Could you check a few things on this model? Use its own coordinates, in mm. Face numbers are marked on the shaded views. A direction names the side the tool comes from. Round coordinates to 2 decimals unless told otherwise and drop trailing zeros. Loops run counter-clockwise (first coordinate to the right, second up) from the corner with the lowest first, then second, coordinate; pieces in that order, holes last. Notation, with made-up numbers: M 5,33 L 12,33 A19 cw 12,38 Z; hole C 32.25,21 d11. An arc over 180 degrees is marked long. One line per item, written item: value. Start each with the question number.
Q1. Which directions (+Z, -Z, +X, -X, +Y, -Y) give clear straight access to the entire face, cutting with the end or side of a thin tool? Please do the marked faces 1, 2 and 3.
Q2. Imagine slicing it at B-B (z = -8). Please give me the cut outline in (x, y).
Q3. I'm going to push flat-ended pins straight in: pin 1 Ø4 at (x, y) = (-72.86, 11.88) entering from -Z (1 decimal); pin 2 Ø4 at (x, z) = (-1, 0.5) entering from -Y; pin 3 Ø6 at (x, y) = (-41.11, 11.88) entering from -Z; pin 4 Ø1 at (y, z) = (0, 17) entering from -X. Where does each tip first touch, or does it pass through?
Q4. Please list where these lines run through material, in increasing order: line 1 along X through (y, z) = (-2.75, -8); line 2 along X through (y, z) = (-2, 0); line 3 along Y through (x, z) = (-7, 3).
Q5. Imagine slicing it at C-C (y = 15.5). Please give me the cut outline in (x, z), then the cut area to 3 significant figures.
Q6. Imagine slicing it at D-D (x = -62.5). Please give me the cut outline in (y, z) (3 decimals), then the cut area to 3 significant figures.
Q7. Imagine slicing it at A-A (y = -4). Give the number of separate pieces and of enclosed holes in the cut face, then the cut area to 3 significant figures.
from build123d import *

# Parameters (mm, degrees)
SKETCH6_W                = 9.525
SKETCH6_H                = 25.4
BOSS_EXTRUDE1_DEPTH      = 8
SKETCH16_W               = 8
SKETCH16_H               = 23
BOSS_EXTRUDE6_DEPTH      = 8
SKETCH7_R                = 3
SKETCH7_R_2              = 2.4
CUT_EXTRUDE1_DEPTH       = 0.8
SKETCH7_3_R              = 2.4
CUT_EXTRUDE2_DEPTH       = 7.2
SKETCH9_R                = 3
CUT_EXTRUDE4_DEPTH       = 0.8
BOSS_EXTRUDE3_DEPTH      = 8
FILLET1_R                = 3.175
FILLET3_R                = 3.175
BOSS_EXTRUDE7_DEPTH      = 18.225
BOSS_EXTRUDE7_DEPTH_BACK = 26.225
SKETCH18_W               = 44.45
SKETCH18_H               = 6.35
FILLET6_R                = 12.7
FILLET7_R                = 6.35
SKETCH11_W               = 8
SKETCH11_H               = 23
BOSS_EXTRUDE4_DEPTH      = 6.746167864
SKETCH14_W               = 8
SKETCH14_H               = 23
BOSS_EXTRUDE5_DEPTH      = 3.6
SKETCH13_R               = 3.1
SKETCH13_R_2             = 2.4
CUT_EXTRUDE5_DEPTH       = 0.8
CUT_EXTRUDE6_START       = -8
CUT_EXTRUDE6_OUTLINE_R   = 2.4
CUT_EXTRUDE6_DEPTH       = 8
F_8_CLEARANCE_HOLE1_D    = 4.4958
FILLET8_R                = 3.175


# Read off the part's stored shape, not the designer's step: Cut-Extrude6
with BuildPart() as part:
    # Sketch6 → Boss-Extrude1 (new body)
    with BuildSketch(Plane(origin=(0, 0, 0), x_dir=(1, 0, 0), z_dir=(0, 1, 0))):
        Rectangle(SKETCH6_W, SKETCH6_H)
    extrude(amount=-BOSS_EXTRUDE1_DEPTH)

    # Sketch16 → Boss-Extrude6 (add)
    with BuildSketch(Plane.XZ):
        with Locations((-6.442250006, 5.512369214)):
            Rectangle(SKETCH16_W, SKETCH16_H)
    extrude(amount=BOSS_EXTRUDE6_DEPTH)

    # Sketch7 → Cut-Extrude1 (cut)
    # profile 1 of 3: a face of its own
    with BuildSketch(Plane(origin=(0, 0, 0), x_dir=(1, 0, 0), z_dir=(0, 1, 0))):
        with Locations(Location((0, 8, 0), (0, 0, 270))):
            Circle(SKETCH7_R)
        with Locations(Location((0, 8, 0), (0, 0, 270))):
            Circle(SKETCH7_R_2, mode=Mode.SUBTRACT)
    # profile 2 of 3: a face of its own
    with BuildSketch(Plane(origin=(0, 0, 0), x_dir=(1, 0, 0), z_dir=(0, 1, 0))):
        with Locations(Location((0, 0, 0), (0, 0, 270))):
            Circle(SKETCH7_R)
        with Locations(Location((0, 0, 0), (0, 0, 270))):
            Circle(SKETCH7_R_2, mode=Mode.SUBTRACT)
    # profile 3 of 3: a face of its own
    with BuildSketch(Plane(origin=(0, 0, 0), x_dir=(1, 0, 0), z_dir=(0, 1, 0))):
        with Locations(Location((0, -8, 0), (0, 0, 270))):
            Circle(SKETCH7_R)
        with Locations(Location((0, -8, 0), (0, 0, 270))):
            Circle(SKETCH7_R_2, mode=Mode.SUBTRACT)
    extrude(amount=-CUT_EXTRUDE1_DEPTH, mode=Mode.SUBTRACT)

    # Sketch7<3> → Cut-Extrude2 (cut)
    with BuildSketch(Plane(origin=(0, 0, 0), x_dir=(1, 0, 0), z_dir=(0, 1, 0))):
        with Locations(Location((0, 8, 0), (0, 0, 270))):
            Circle(SKETCH7_3_R)
        with Locations(Location((0, 0, 0), (0, 0, 270))):
            Circle(SKETCH7_3_R)
        with Locations(Location((0, -8, 0), (0, 0, 270))):
            Circle(SKETCH7_3_R)
    extrude(amount=-CUT_EXTRUDE2_DEPTH, mode=Mode.SUBTRACT)

    # Sketch9 → Cut-Extrude4 (cut)
    with BuildSketch(Plane(origin=(0, -7.2, -7.2), x_dir=(1, 0, 0), z_dir=(0, 1, 0))):
        with Locations(Location((0, 0.8, 0), (0, 0, 270))):
            Circle(SKETCH9_R)
        with Locations(Location((0, -7.2, 0), (0, 0, 270))):
            Circle(SKETCH9_R)
        with Locations(Location((0, -15.2, 0), (0, 0, 270))):
            Circle(SKETCH9_R)
    extrude(amount=-CUT_EXTRUDE4_DEPTH, mode=Mode.SUBTRACT)

    # Sketch10 → Boss-Extrude3 (add)
    with BuildSketch(Plane(origin=(0, -8, 0), x_dir=(-1, 0, 0), z_dir=(0, -1, 0))):
        Polygon((4.7625, 4.223850374), (34.7625, -22.098), (60.1625, -22.098), (60.1625, -28.448), (32.37167179, -28.448), (4.7625, -4.223850374), align=None)
    extrude(amount=-BOSS_EXTRUDE3_DEPTH)

    # Fillet1
    fillet1_edges = [part.edges().sort_by_distance(p)[0] for p in [
        (-2.442250006, -4, 12.7),
        (-4.7625, -4, -5.987630786),
    ]]
    fillet(fillet1_edges, radius=FILLET1_R)

    # Fillet3
    fillet3_edges = [part.edges().sort_by_distance(p)[0] for p in [
        (4.7625, -4, 12.7),
        (-4.7625, -4, -12.7),
        (4.7625, -4, -12.7),
    ]]
    fillet(fillet3_edges, radius=FILLET3_R)

    # Sketch18 → Boss-Extrude7 (add, two sides: drawn at the far end of the back side and taken through both)
    with BuildSketch(Plane(origin=(0, 0, 0), x_dir=(1, 0, 0), z_dir=(0, 1, 0)).offset(-BOSS_EXTRUDE7_DEPTH_BACK)):
        with Locations((-56.9875, -25.273)):
            Rectangle(SKETCH18_W, SKETCH18_H)
    extrude(amount=BOSS_EXTRUDE7_DEPTH + BOSS_EXTRUDE7_DEPTH_BACK)

    # Fillet6
    fillet6_edges = [part.edges().sort_by_distance(p)[0] for p in [
        (-32.37167179, -4, 28.448),
    ]]
    fillet(fillet6_edges, radius=FILLET6_R)

    # Fillet7
    fillet7_edges = [part.edges().sort_by_distance(p)[0] for p in [
        (-34.7625, -4, 22.098),
    ]]
    fillet(fillet7_edges, radius=FILLET7_R)

    # Sketch11 → Boss-Extrude4 (add)
    with BuildSketch(Plane(origin=(0, -8, 0), x_dir=(-1, 0, 0), z_dir=(0, -1, 0))):
        with Locations((6.44225, -5.512369144)):
            Rectangle(SKETCH11_W, SKETCH11_H)
    extrude(amount=BOSS_EXTRUDE4_DEPTH)

    # Sketch14 → Boss-Extrude5 (add)
    with BuildSketch(Plane(origin=(0, -14.746167864, 0), x_dir=(-1, 0, 0), z_dir=(0, -1, 0))):
        with Locations((6.44225, -5.512369144)):
            Rectangle(SKETCH14_W, SKETCH14_H)
    extrude(amount=BOSS_EXTRUDE5_DEPTH)

    # Sketch13 → Cut-Extrude5 (cut)
    # profile 1 of 3: a face of its own
    with BuildSketch(Plane(origin=(-2.442250006, 0, 0), x_dir=(0, 0, -1), z_dir=(1, 0, 0))):
        with Locations((-13.512369144, -14.746167864)):
            Circle(SKETCH13_R)
        with Locations((-13.512369144, -14.746167864)):
            Circle(SKETCH13_R_2, mode=Mode.SUBTRACT)
    # profile 2 of 3: a face of its own
    with BuildSketch(Plane(origin=(-2.442250006, 0, 0), x_dir=(0, 0, -1), z_dir=(1, 0, 0))):
        with Locations((2.487630856, -14.746167864)):
            Circle(SKETCH13_R)
        with Locations((2.487630856, -14.746167864)):
            Circle(SKETCH13_R_2, mode=Mode.SUBTRACT)
    # profile 3 of 3: a face of its own
    with BuildSketch(Plane(origin=(-2.442250006, 0, 0), x_dir=(0, 0, -1), z_dir=(1, 0, 0))):
        with BuildLine():
            Line((-6.312369144, -14.014797014), (-6.312369144, -12.552055314))
            ThreePointArc((-6.312369144, -12.552055314), (-5.512369144, -12.425918689), (-4.712369144, -12.552055314))
            Line((-4.712369144, -12.552055314), (-4.712369144, -14.014797014))
            Line((-4.712369144, -14.014797014), (-3.249627444, -14.014797014))
            ThreePointArc((-3.249627444, -14.014797014), (-3.144641809, -14.746167864), (-3.249627444, -15.477538714))
            Line((-3.249627444, -15.477538714), (-4.712369144, -15.477538714))
            Line((-4.712369144, -15.477538714), (-4.712369144, -16.940280414))
            ThreePointArc((-4.712369144, -16.940280414), (-5.512369144, -17.066417039), (-6.312369144, -16.940280414))
            Line((-6.312369144, -16.940280414), (-6.312369144, -15.477538714))
            Line((-6.312369144, -15.477538714), (-7.775110844, -15.477538714))
            ThreePointArc((-7.775110844, -15.477538714), (-7.880096479, -14.746167864), (-7.775110844, -14.014797014))
            Line((-7.775110844, -14.014797014), (-6.312369144, -14.014797014))
        make_face()
    cut_extrude5 = extrude(amount=-CUT_EXTRUDE5_DEPTH, mode=Mode.SUBTRACT)

    # Cut-Extrude6 outline → Cut-Extrude6 (cut)
    with BuildSketch(Plane(origin=(-2.442250006, 0, 0), x_dir=(0, 0, -1), z_dir=(1, 0, 0)).offset(CUT_EXTRUDE6_START)):
        with BuildLine():
            Line((-4.712369144, -15.477538714), (-3.249627444, -15.477538714))
            ThreePointArc((-3.249627444, -15.477538714), (-3.144641809, -14.746167864), (-3.249627444, -14.014797014))
            Line((-3.249627444, -14.014797014), (-4.712369144, -14.014797014))
            Line((-4.712369144, -14.014797014), (-4.712369144, -12.552055314))
            ThreePointArc((-4.712369144, -12.552055314), (-5.512369144, -12.425918689), (-6.312369144, -12.552055314))
            Line((-6.312369144, -12.552055314), (-6.312369144, -14.014797014))
            Line((-6.312369144, -14.014797014), (-7.775110844, -14.014797014))
            ThreePointArc((-7.775110844, -14.014797014), (-7.880096479, -14.746167864), (-7.775110844, -15.477538714))
            Line((-7.775110844, -15.477538714), (-6.312369144, -15.477538714))
            Line((-6.312369144, -15.477538714), (-6.312369144, -16.940280414))
            ThreePointArc((-6.312369144, -16.940280414), (-5.512369144, -17.066417039), (-4.712369144, -16.940280414))
            Line((-4.712369144, -16.940280414), (-4.712369144, -15.477538714))
        make_face()
        with Locations((-13.512369144, -14.746167864)):
            Circle(CUT_EXTRUDE6_OUTLINE_R)
        with Locations((2.487630856, -14.746167864)):
            Circle(CUT_EXTRUDE6_OUTLINE_R)
    extrude(amount=CUT_EXTRUDE6_DEPTH, mode=Mode.SUBTRACT)

    # Mirror1: Cut-Extrude5 across plane
    add(cut_extrude5.mirror(Plane(origin=(-6.442250006, 0, 0), x_dir=(0, 0, 1), z_dir=(1, 0, 0))), mode=Mode.SUBTRACT)

    # #8 Clearance Hole1 (through all)
    with Locations(Plane(origin=(0, 0, 22.098), x_dir=(-1, 0, 0), z_dir=(0, 0, -1))):
        with Locations((72.8625, 11.875), (41.1125, 11.875), (41.1125, -19.875), (72.8625, -19.875)):
            Hole(F_8_CLEARANCE_HOLE1_D / 2)

    # Fillet8
    fillet8_edges = [part.edges().sort_by_distance(p)[0] for p in [
        (-6.44225, -18.346167864, 17.012369144),
        (-6.44225, -18.346167864, -5.987630856),
    ]]
    fillet(fillet8_edges, radius=FILLET8_R)


solid = part.part
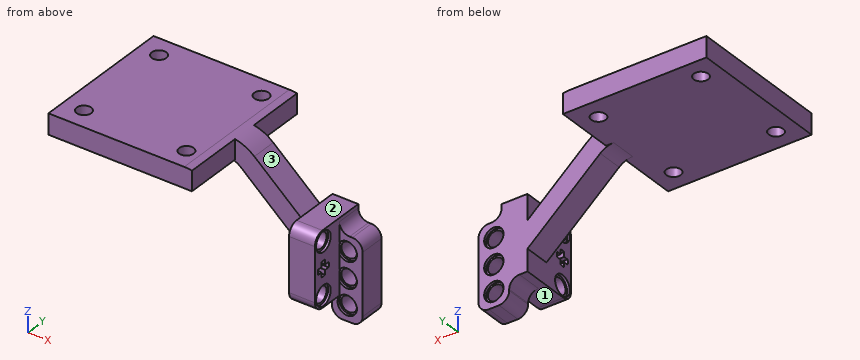
Report:
1. face 1: -Z, -X, -Y
1. face 2: +Z, +X, +Y, -Y
1. face 3: +Z, +Y, -Y
2. outline: M -4.98,-8 L -3,-8 L -3,-7.2 L -2.4,-7.2 L -2.4,-0.8 L -3,-0.8 L -3,0 L -4.98,0 Z; M 2.4,-7.2 L 3,-7.2 L 3,-8 L 4.76,-8 L 4.76,0 L 3,0 L 3,-0.8 L 2.4,-0.8 Z
3. pin 1: passes through
3. pin 2: stops at y = -18.35
3. pin 3: stops at z = 22.1
3. pin 4: stops at x = -29.52
4. line 1: x = -4.98 to -2.4, 2.4 to 4.76
4. line 2: x = -10.44 to -2.4, 2.4 to 4.76
4. line 3: y = -18.35 to 0
5. outline: M -79.21,22.1 L -34.76,22.1 L -34.76,28.22 A12.7 ccw -37.15,28.45 L -79.21,28.45 Z
5. area: 282 mm²
6. outline: M -26.225,22.098 L 18.225,22.098 L 18.225,28.448 L -26.225,28.448 Z
6. area: 282 mm²
7. separate pieces: 1
7. enclosed holes: 3
7. area: 809 mm²
